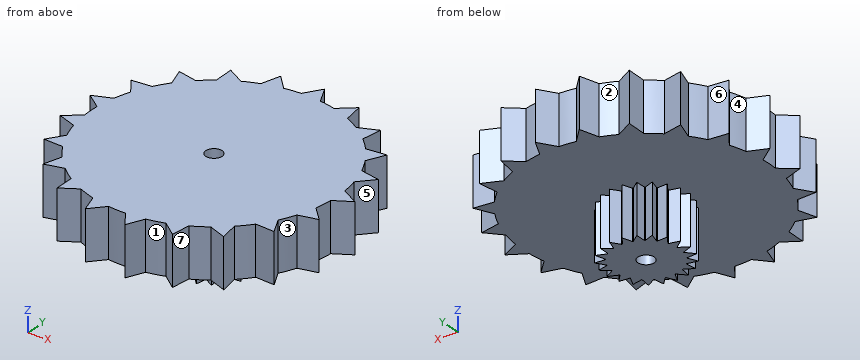
```python
from build123d import *

# Parameters (mm, degrees)
BOSS_EXTRUDE1_DEPTH = 3
BOSS_EXTRUDE3_DEPTH = 3
CIRPATTERN1_COUNT   = 21
SKETCH7_R           = 2
BOSS_EXTRUDE4_DEPTH = 3
BOSS_EXTRUDE5_DEPTH = 3
CIRPATTERN2_COUNT   = 21
SKETCH9_R           = 0.5
CUT_EXTRUDE1_DEPTH  = 6


with BuildPart() as part:
    # Sketch3 → Boss-Extrude1 (new body)
    with BuildSketch(Plane(origin=(0, 0, -25.970633743), x_dir=(-1, 0, 0), z_dir=(0, 0, -1))):
        with BuildLine():
            ThreePointArc((-1.041352606, 75.627353819), (0.431341592, 60.712413978), (0.181550718, 75.6978023))
            Line((0.181550718, 75.6978023), (-1.041352606, 75.627353819))
        make_face()
    extrude(amount=BOSS_EXTRUDE1_DEPTH)

    # Sketch5 → Boss-Extrude3 (add)
    with BuildSketch(Plane.XY.offset(-25.970633743)):
        Polygon((-0.181550718, 75.6978023), (1.041352606, 75.627353819), (0.491951555, 76.73970416), align=None)
    boss_extrude3 = extrude(amount=-BOSS_EXTRUDE3_DEPTH)

    # CirPattern1: Boss-Extrude3 ×21 about axis
    cirpattern1_axis = Axis((0.001629139, 68.228279947, 0), (0, 0, 1))
    for i in range(1, CIRPATTERN1_COUNT):
        add(boss_extrude3.rotate(cirpattern1_axis, i * 360 / CIRPATTERN1_COUNT))

    # Sketch7 → Boss-Extrude4 (add)
    with BuildSketch(Plane(origin=(0, 0, -28.970633743), x_dir=(-1, 0, 0), z_dir=(0, 0, -1))):
        with Locations((0, 68.2)):
            Circle(SKETCH7_R)
    extrude(amount=BOSS_EXTRUDE4_DEPTH)

    # Sketch8 → Boss-Extrude5 (add)
    with BuildSketch(Plane(origin=(0, 0, -31.970633743), x_dir=(-1, 0, 0), z_dir=(0, 0, -1))):
        Polygon((0.4, 66.4), (-0.4, 66.4), (0, 65.6), align=None)
    boss_extrude5 = extrude(amount=-BOSS_EXTRUDE5_DEPTH)

    # CirPattern2: Boss-Extrude5 ×21 about axis
    cirpattern2_axis = Axis((0, 68.168195033, 0), (0, 0, 1))
    for i in range(1, CIRPATTERN2_COUNT):
        add(boss_extrude5.rotate(cirpattern2_axis, i * 360 / CIRPATTERN2_COUNT))

    # Sketch9 → Cut-Extrude1 (cut)
    with BuildSketch(Plane(origin=(0, 0, -31.970633743), x_dir=(-1, 0, 0), z_dir=(0, 0, -1))):
        with Locations((0, 68.2)):
            Circle(SKETCH9_R)
    extrude(amount=-CUT_EXTRUDE1_DEPTH, mode=Mode.SUBTRACT)


solid = part.part
```
Source: CAD feature listing. Evaluate the final solid. Frame: model axes, mm. Face numbers are marked on the shaded views. A direction names the side the tool comes from. Round coordinates to 2 decimals unless told otherwise and drop trailing zeros. Use CSV: the item, a comma, the result in double quotes.
Q1. Ray query, line 1 along Z through (x, y) = (4, 72); line 2 along X through (y, z) = (68.2, -27.7); line 3 along Y through (x, z) = (1.75, -27.05). Return the intervals inside material, ascending.
Reported:
line 1,"-28.97 to -25.97"
line 2,"-7.5 to -0.5, 0.5 to 8.23"
line 3,"60.91 to 75.49"
Q2. Pin query (flat end, axial travel): pin 1 Ø3 at (y, z) = (73.5, -27) entering from +X; pin 2 Ø3 at (y, z) = (71, -28) entering from +X; pin 3 Ø3 at (x, z) = (-5, -27) entering from -Y. Return the tip coordinate at first contact, or that it passes through.
Reported:
pin 1,"x = 6.96"
pin 2,"x = 8.1"
pin 3,"y = 60.77"
Q3. Reachability of the marked faces 1, 2, 3 and 4 from +Z, -Z, +X, -X, +Y, -Y: full face, straight path, thin tool, end or side. Return the list, or none.
Reported:
face 1,"+Z, -Z, -Y"
face 2,"+Z, -Z, +Y"
face 3,"+Z, -Z, +X"
face 4,"+Z, -Z, -X"
Q4. Mould query, pull axis Y, two halves, no side actions, for the marked faces 5, 6 and 7. Classes: pulls with the +Y half, pulls with the -Y half, needs draft (parallel to the pull), parting line crosses it, or undercut.
Reported:
face 5,"undercut"
face 6,"pulls with the +Y half"
face 7,"pulls with the -Y half"
